Design review of the part built by this model. Coordinates are the model's own, in mm. A direction names the side the tool comes from. Round coordinates to 2 decimals unless told otherwise and drop trailing zeros. Order: outer loops, then holes, each group sorted by start corner. A loop starts at its lowest first (then second) coordinate and runs counter-clockwise, first axis right, second up. Notation, with made-up numbers: M 67,19.25 L 103,19.25 A31 ccw 103,56.25 Z; hole C 80.5,41.25 d1. An arc over 180 degrees is marked long. Write item = value, one per line. Start each with the question number.
```python
from build123d import *

# Parameters (mm, degrees)
BOSS_EXTRUDE2_DEPTH = 30
SKETCH2_R           = 1.25
CUT_EXTRUDE1_DEPTH  = 10
SKETCH4_R           = 2
CUT_EXTRUDE5_DEPTH  = 37.400549446
SKETCH5_R           = 3.05
CUT_EXTRUDE6_DEPTH  = 2.7


with BuildPart() as part:
    # Sketch1 → Boss-Extrude2 (new body)
    with BuildSketch(Plane(origin=(0, 0, 0), x_dir=(1, 0, 0), z_dir=(0, 1, 0))):
        Polygon((0, 0), (-20, 0), (-20, 5), (-11, 5), (-5.01141852, 10), (5.01141852, 10), (11, 5), (20, 5), (20, 0), align=None)
    extrude(amount=BOSS_EXTRUDE2_DEPTH)

    # Sketch2 → Cut-Extrude1 (cut)
    with BuildSketch(Plane(origin=(0, 30, 0), x_dir=(1, 0, 0), z_dir=(0, 1, 0))):
        with Locations(Location((0, 4, 0), (0, 0, 270))):
            Circle(SKETCH2_R)
    extrude(amount=-CUT_EXTRUDE1_DEPTH, mode=Mode.SUBTRACT)

    # Sketch4 → Cut-Extrude5 (cut, through all)
    with BuildSketch(Plane(origin=(0, 0, -5), x_dir=(-1, 0, 0), z_dir=(0, 0, -1))):
        with Locations((-15.5, 4)):
            Circle(SKETCH4_R)
        with Locations(Location((-15.5, 26, 0), (0, 0, 180))):
            Circle(SKETCH4_R)
        with Locations(Location((15.5, 4, 0), (0, 0, 180))):
            Circle(SKETCH4_R)
        with Locations((15.5, 26)):
            Circle(SKETCH4_R)
    extrude(amount=-CUT_EXTRUDE5_DEPTH, mode=Mode.SUBTRACT)

    # Sketch5 → Cut-Extrude6 (cut)
    with BuildSketch(Plane(origin=(0, 30, 0), x_dir=(1, 0, 0), z_dir=(0, 1, 0))):
        with Locations(Location((0, 4, 0), (0, 0, 270))):
            Circle(SKETCH5_R)
    extrude(amount=-CUT_EXTRUDE6_DEPTH, mode=Mode.SUBTRACT)


solid = part.part
```
(1) Draft analysis for pull direction Z (two halves, no side actions). For faces 5 (the face through (0.05, 23.7, -5.25)), 6 (the face through (7.96, 14.79, -7.54)), 7 (the face through (0, 0, -4)), state which applies: pulls with the +Z half, pulls with the -Z half, needs draft (parallel to the pull), parting line crosses it, or undercut.
(2) For line 1 along Y through (x, z) = (-15.5, -2.4); line 2 along Z through (x, y) = (13, 25.25); line 3 along Y through (x, z) = (3, -4), list the stretches that pass through material, from the lowest coordinate up. Write a range as [from, to].
(3) Insertion check: pin 1 (2 mm diameter, centred on y = 16.5, z = -7, fed in from +X); pin 2 (5 mm diameter, centred on x = 0, z = -3.5, fed in from +Y); pin 3 (10 mm diameter, centred on x = -14.5, y = 19.5, fed in from -Z). Each pin has a flat end and moves straight along its axis. Give the tip position at first contact, or say it passes through.
(4) Consider section D-D, the plane y = 4. Write out the cut boundary in (x, z).
(5) Consider section A-A, the plane y = 26. Write out the cut boundary in (x, z), then the cut area to 3 significant figures.
(6) For faces 1 (the face through (13.9, 27.2, -2.5)), 2 (the face through (15, 15, -5)), 3 (the face through (-16, 15, -5)), 4 (the face through (-1, 27.3, -3)), list the 3-axis set-ups (+Z, -Z, +X, -X, +Y, -Y) from which the entire face can be reached by the end or side of a thin tool; tool diameter is ignored.
(7) Consider section C-C, the plane z = -4. Write out the cut boundary in (x, y), then the cut area to 3 significant figures.
(8) Consider section B-B, the plane x = -15.5. Write out the cut boundary in (y, z).
Completed:
q1.face_5 = undercut
q1.face_6 = pulls with the -Z half
q1.face_7 = needs draft
q2.line_1 = [0, 2], [6, 24], [28, 30]
q2.line_2 = [-5, 0]
q2.line_3 = [0, 27.3]
q3.pin_1 = 9.8
q3.pin_2 = 27.3
q3.pin_3 = -6.25
q4.outline = M -20,-5 L -17.5,-5 L -17.5,0 L -20,0 Z; M -13.5,-5 L -11,-5 L -5.01,-10 L 5.01,-10 L 11,-5 L 13.5,-5 L 13.5,0 L -13.5,0 Z; M 17.5,-5 L 20,-5 L 20,0 L 17.5,0 Z
q5.outline = M -20,-5 L -17.5,-5 L -17.5,0 L -20,0 Z; M -13.5,-5 L -11,-5 L -5.01,-10 L 5.01,-10 L 11,-5 L 13.5,-5 L 13.5,0 L -13.5,0 Z; M 17.5,-5 L 20,-5 L 20,0 L 17.5,0 Z; hole C 0,-4 d2.5
q5.area = 235 mm2
q6.face_1 = +Z, -Z
q6.face_2 = -Z, +X, +Y, -Y
q6.face_3 = -Z, -X, +Y, -Y
q6.face_4 = +Y
q7.outline = M -20,0 L 20,0 L 20,30 L 3.05,30 L 3.05,27.3 L 1.25,27.3 L 1.25,20 L -1.25,20 L -1.25,27.3 L -3.05,27.3 L -3.05,30 L -20,30 Z; hole C -15.5,4 d4; hole C -15.5,26 d4; hole C 15.5,4 d4; hole C 15.5,26 d4
q7.area = 1,120 mm2
q8.outline = M 0,-5 L 2,-5 L 2,0 L 0,0 Z; M 6,-5 L 24,-5 L 24,0 L 6,0 Z; M 28,-5 L 30,-5 L 30,0 L 28,0 Z
